from build123d import *

# Parameters (mm, degrees)
F0_R           = 16
F1_DEPTH       = 50
F2_R           = 16
F3_DEPTH       = 20
F2_W           = 60
F2_H           = 10
F4_DEPTH       = 50
F6_DEPTH       = 20
F6_DEPTH_BACK  = 10
F7_DEPTH       = 20
F7_DEPTH_BACK  = 10
F8_DEPTH       = 10
F9_R           = 5
F10_R          = 5
F12_DEPTH      = 15
F12_DEPTH_BACK = 14.9
F13_R          = 3


with BuildPart() as f1:
    # F0 (on Top) → F1 (new body)
    with BuildSketch(Plane.XY):
        Circle(F0_R)
    extrude(amount=F1_DEPTH)

    # F2 (on face) → F3 (join)
    with BuildSketch(Plane.XY.offset(50)):
        Polygon((-30, 22.5), (-30, 0), (-30, -32.5), (30, -32.5), (30, 0), (30, 22.5), align=None)
        Circle(F2_R, mode=Mode.SUBTRACT)
        Circle(F2_R)
    extrude(amount=F3_DEPTH)

    # F2 (on face) → F4 (join)
    with BuildSketch(Plane.XY.offset(50)):
        with Locations((0, 27.5)):
            Rectangle(F2_W, F2_H)
    extrude(amount=F4_DEPTH)

    # F5 (on face) → F6 (cut, two sides)
    with BuildSketch(Plane.XZ.offset(-22.5)) as f6_sk:
        with BuildLine():
            ThreePointArc((-6, 100), (0, 94), (6, 100))
            Line((6, 100), (-6, 100))
        make_face()
        with BuildLine():
            Line((-6, 100), (6, 100))
            ThreePointArc((6, 100), (0, 106), (-6, 100))
        make_face()
    extrude(amount=F6_DEPTH, mode=Mode.SUBTRACT)
    extrude(f6_sk.sketch, amount=-F6_DEPTH_BACK, mode=Mode.SUBTRACT)

    # F5 (on face) → F7 (join, two sides)
    with BuildSketch(Plane.XZ.offset(-22.5)) as f7_sk:
        with BuildLine():
            ThreePointArc((-10, 100), (0, 90), (10, 100))
            Line((10, 100), (6, 100))
            ThreePointArc((6, 100), (0, 94), (-6, 100))
            Line((-6, 100), (-10, 100))
        make_face()
        with BuildLine():
            Line((6, 100), (10, 100))
            ThreePointArc((10, 100), (0, 110), (-10, 100))
            Line((-10, 100), (-6, 100))
            ThreePointArc((-6, 100), (0, 106), (6, 100))
        make_face()
    extrude(amount=F7_DEPTH)
    extrude(f7_sk.sketch, amount=-F7_DEPTH_BACK)

    # F5 (on face) → F8 (join)
    with BuildSketch(Plane.XZ.offset(-22.5)):
        with BuildLine():
            Line((10, 100), (30, 100))
            ThreePointArc((30, 100), (0, 130), (-30, 100))
            Line((-30, 100), (-10, 100))
            ThreePointArc((-10, 100), (0, 110), (10, 100))
        make_face()
    extrude(amount=-F8_DEPTH)

    # F9
    f9_edges = [f1.edges().sort_by_distance(p)[0] for p in [
        (30, -32.5, 60),
    ]]
    fillet(f9_edges, radius=F9_R)

    # F10
    f10_edges = [f1.edges().sort_by_distance(p)[0] for p in [
        (-30, -32.5, 60),
    ]]
    fillet(f10_edges, radius=F10_R)

    # F11 (on Right) → F12 (cut, two sides)
    with BuildSketch(Plane.YZ) as f12_sk:
        Polygon((6.397780925, 70.0798109174), (-32.611630857, 70.0798109174), (-32.611630857, 59.6272705332), align=None)
    extrude(amount=-F12_DEPTH, mode=Mode.SUBTRACT)
    extrude(f12_sk.sketch, amount=F12_DEPTH_BACK, mode=Mode.SUBTRACT)

    # F13
    f13_edges = [f1.edges().sort_by_distance(p)[0] for p in [
        (-16, 0, 0),
    ]]
    fillet(f13_edges, radius=F13_R)


solid = f1.part
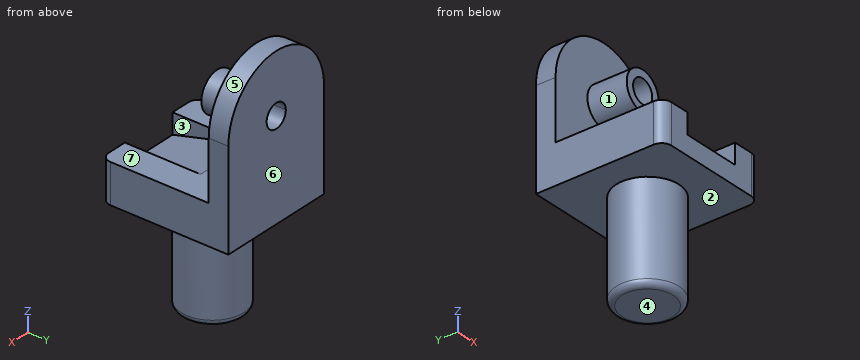
Build history of the part. All positions in model axes, mm. Face numbers are marked on the shaded views. A direction names the side the tool comes from. Round coordinates to 2 decimals unless told otherwise and drop trailing zeros. Write each loop counter-clockwise with the first axis right and the second up, starting at its lowest first coordinate (ties: lowest second). Pieces come first, ordered by that corner, then holes. Notation, with made-up numbers: M -12,-3.75 L 45,-3.75 A24 cw 45,9.25 Z; hole C -11.5,38.25 d3. An arc over 180 degrees is marked long. Answer in a Markdown table with one row per item.
1. Flat gauge pins, fed straight in: P1, Ø10, axis at x = -7.5, y = -2, coming from the +Z side; P2, Ø12, axis at x = 9.5, y = -8.5, coming from the +Z side; P3, Ø16, axis at x = 4, z = 96, coming from the -Y side; P4, Ø11, axis at x = 0, z = 100, coming from the -Y side. Where does each tip first touch, or does it go through?
Geometry check:
| item | result |
|---|---|
| P1 | z = 108.47 |
| P2 | z = 70 |
| P3 | y = 2.5 |
| P4 | through |
2. Probe L1, parallel to Z at x = 0, y = 10; L2, parallel to Z at x = 0, y = 18.5; L3, parallel to X at y = 9, z = 100. List the from-to ranges inside material, lowest first. Write a range as [from, to].
Geometry check:
| item | result |
|---|---|
| L1 | [0, 70], [90, 94], [106, 110] |
| L2 | [50, 70], [90, 94], [106, 110] |
| L3 | [-10, -6], [6, 10] |
3. Mould opens along Z. For the marked faces 4, 5, 6 and 7 say: +Z half, -Z half, draft (parallel to the pull), parting line (faces both ways), or undercut.
Geometry check:
| item | result |
|---|---|
| face 4 | -Z half |
| face 5 | +Z half |
| face 6 | draft |
| face 7 | undercut |
4. Saw through at B-B (z = 61). List the corners of the cut face in (x, y).
Geometry check:
| item | result |
|---|---|
| outline | M -30,-27.5 A5 ccw -25,-32.5 L -15,-32.5 L -15,-27.49 L 14.9,-27.49 L 14.9,-32.5 L 25,-32.5 A5 ccw 30,-27.5 L 30,32.5 L -30,32.5 Z |
5. Saw through at A-A (x = 0). List the corners of the cut face in (y, z), and give its area (3 significant figures).
Geometry check:
| item | result |
|---|---|
| outline | M -32.5,50 L -16,50 L -16,3 A3 ccw -13,0 L 13,0 A3 ccw 16,3 L 16,50 L 32.5,50 L 32.5,94 L 2.5,94 L 2.5,90 L 22.5,90 L 22.5,70 L 6.1,70 L -32.5,59.66 Z; M 2.5,106 L 32.5,106 L 32.5,130 L 22.5,130 L 22.5,110 L 2.5,110 Z |
| area | 3,340 mm2 |
6. Which spindle directions (+Z, -Z, +X, -X, +Y, -Y) get a long thin tool onto all of the face, cutting with end or side? Do the marked faces 1, 2 and 3. Say none if no direction does.
Geometry check:
| item | result |
|---|---|
| face 1 | -Y |
| face 2 | -Z |
| face 3 | +Z, -Y |
7. Saw through at C-C (y = -26). List the corners of the cut face in (x, z), and give its area (3 significant figures).
Geometry check:
| item | result |
|---|---|
| outline | M -30,50 L 30,50 L 30,70 L 14.9,70 L 14.9,61.4 L -15,61.4 L -15,70 L -30,70 Z |
| area | 943 mm2 |
8. Saw through at D-D (y = 4). State how many separate pieces and enclosed holes the cut face has, and give its area (3 significant figures).
Geometry check:
| item | result |
|---|---|
| separate pieces | 2 |
| enclosed holes | 1 |
| area | 2,930 mm2 |
